CAD build for the part. Positions are in the model's coordinates, mm. Give positions to 0.01 mm unless a question says otherwise; leave off trailing zeros. Loops run counter-clockwise (first coordinate to the right, second up) from the corner with the lowest first, then second, coordinate; pieces in that order, holes last.
```python
from build123d import *

# Parameters (mm, degrees)
SKETCH1_R               = 25
BOSS_EXTRUDE1_DEPTH     = 3.5
SKETCH3_R               = 8.75
BOSS_EXTRUDE2_DEPTH     = 4
SKETCH4_R               = 2.625
CUT_EXTRUDE1_DEPTH      = 3.5
CUT_EXTRUDE2_DEPTH      = 10
CUT_EXTRUDE3_DEPTH      = 26
CUT_EXTRUDE3_DEPTH_BACK = 26
CUT_EXTRUDE4_DEPTH      = 26
CUT_EXTRUDE4_DEPTH_BACK = 26
SKETCH11_R              = 25
CUT_EXTRUDE5_DEPTH      = 3
BOSS_EXTRUDE3_DEPTH     = 3
SKETCH13_R              = 8.75
SKETCH13_R_2            = 2.55
BOSS_EXTRUDE4_DEPTH     = 3
SKETCH16_R              = 25
SKETCH16_R_2            = 2.625
BOSS_EXTRUDE5_DEPTH     = 2.5
SKETCH17_R              = 25
SKETCH17_R_2            = 8.75
CUT_EXTRUDE6_DEPTH      = 0.75
CUT_EXTRUDE7_DEPTH      = 1
SKETCH19_R              = 8.75
SKETCH19_R_2            = 3.5
CUT_EXTRUDE8_DEPTH      = 20
SKETCH20_R              = 6.415433717
CUT_EXTRUDE9_DEPTH      = 10
SKETCH22_R              = 3.5
CUT_EXTRUDE10_DEPTH     = 0.5


with BuildPart() as part:
    # Sketch1 → Boss-Extrude1 (new body)
    with BuildSketch(Plane(origin=(0, 0, 0), x_dir=(1, 0, 0), z_dir=(0, 1, 0))):
        Circle(SKETCH1_R)
    extrude(amount=BOSS_EXTRUDE1_DEPTH)

    # Sketch3 → Boss-Extrude2 (add)
    with BuildSketch(Plane(origin=(0, 3.5, 0), x_dir=(1, 0, 0), z_dir=(0, 1, 0))):
        Circle(SKETCH3_R)
    extrude(amount=BOSS_EXTRUDE2_DEPTH)

    # Sketch4 → Cut-Extrude1 (cut)
    with BuildSketch(Plane(origin=(0, 3.5, 0), x_dir=(1, 0, 0), z_dir=(0, 1, 0))):
        with Locations((0, 18.5)):
            Circle(SKETCH4_R)
        with Locations((13.081475452, 13.081475452)):
            Circle(SKETCH4_R)
        with Locations((18.5, 0)):
            Circle(SKETCH4_R)
        with Locations((13.081475452, -13.081475452)):
            Circle(SKETCH4_R)
        with Locations((0, -18.5)):
            Circle(SKETCH4_R)
        with Locations((-13.081475452, -13.081475452)):
            Circle(SKETCH4_R)
        with Locations((-18.5, 0)):
            Circle(SKETCH4_R)
        with Locations((-13.081475452, 13.081475452)):
            Circle(SKETCH4_R)
    extrude(amount=-CUT_EXTRUDE1_DEPTH, mode=Mode.SUBTRACT)

    # Sketch7 → Cut-Extrude2 (cut)
    with BuildSketch(Plane.XZ):
        with BuildLine():
            Line((1.9, 1.700735135), (1.9, -1.700735135))
            ThreePointArc((1.9, -1.700735135), (-2.55, 0), (1.9, 1.700735135))
        make_face()
    extrude(amount=-CUT_EXTRUDE2_DEPTH, mode=Mode.SUBTRACT)

    # Sketch8 → Cut-Extrude3 (cut, two sides)
    with BuildSketch(Plane(origin=(0, 0, 0), x_dir=(0, 0, -1), z_dir=(1, 0, 0))) as cut_extrude3_sk:
        with BuildLine():
            Line((-2.5, 6), (2.5, 6))
            ThreePointArc((2.5, 6), (3.5, 5), (2.5, 4))
            Line((2.5, 4), (-2.5, 4))
            ThreePointArc((-2.5, 4), (-3.5, 5), (-2.5, 6))
        make_face()
    extrude(amount=CUT_EXTRUDE3_DEPTH, mode=Mode.SUBTRACT)
    extrude(cut_extrude3_sk.sketch, amount=-CUT_EXTRUDE3_DEPTH_BACK, mode=Mode.SUBTRACT)

    # Sketch9 → Cut-Extrude4 (cut, two sides)
    with BuildSketch(Plane.XY) as cut_extrude4_sk:
        with BuildLine():
            Line((-2.5, 6), (2.5, 6))
            ThreePointArc((2.5, 6), (3.5, 5), (2.5, 4))
            Line((2.5, 4), (-2.5, 4))
            ThreePointArc((-2.5, 4), (-3.5, 5), (-2.5, 6))
        make_face()
    extrude(amount=CUT_EXTRUDE4_DEPTH, mode=Mode.SUBTRACT)
    extrude(cut_extrude4_sk.sketch, amount=-CUT_EXTRUDE4_DEPTH_BACK, mode=Mode.SUBTRACT)

    # Sketch11 → Cut-Extrude5 (cut)
    with BuildSketch(Plane(origin=(0, 3.5, 0), x_dir=(1, 0, 0), z_dir=(0, 1, 0))):
        Circle(SKETCH11_R)
    extrude(amount=-CUT_EXTRUDE5_DEPTH, mode=Mode.SUBTRACT)

    # Sketch12 → Boss-Extrude3 (add)
    with BuildSketch(Plane(origin=(0, 0.5, 0), x_dir=(1, 0, 0), z_dir=(0, 1, 0))):
        Polygon((0.6, 0.6), (5, 0.6), (5, -0.6), (0.6, -0.6), (0.6, -5), (-0.6, -5), (-0.6, -0.6), (-5, -0.6), (-5, 0.6), (-0.6, 0.6), (-0.6, 5), (0.6, 5), align=None)
    extrude(amount=BOSS_EXTRUDE3_DEPTH)

    # Sketch13 → Boss-Extrude4 (add)
    with BuildSketch(Plane(origin=(0, 0.5, 0), x_dir=(1, 0, 0), z_dir=(0, 1, 0))):
        Circle(SKETCH13_R)
        Circle(SKETCH13_R_2, mode=Mode.SUBTRACT)
    extrude(amount=BOSS_EXTRUDE4_DEPTH)

    # Sketch15 → Revolve1 (revolve)
    with BuildSketch(Plane.XY):
        Polygon((0, 13.5), (-8.75, 7.5), (0, 7.5), align=None)
    revolve(axis=Axis((0, -5.481339273, 0), (0, 1, 0)))

    # Sketch16 → Boss-Extrude5 (add)
    with BuildSketch(Plane.XZ):
        Circle(SKETCH16_R)
        with Locations((13.081475452, 13.081475452)):
            Circle(SKETCH16_R_2, mode=Mode.SUBTRACT)
        with Locations((0, 18.5)):
            Circle(SKETCH16_R_2, mode=Mode.SUBTRACT)
        with Locations((-13.081475452, 13.081475452)):
            Circle(SKETCH16_R_2, mode=Mode.SUBTRACT)
        with Locations((-18.5, 0)):
            Circle(SKETCH16_R_2, mode=Mode.SUBTRACT)
        with Locations((-13.081475452, -13.081475452)):
            Circle(SKETCH16_R_2, mode=Mode.SUBTRACT)
        with Locations((0, -18.5)):
            Circle(SKETCH16_R_2, mode=Mode.SUBTRACT)
        with Locations((13.081475452, -13.081475452)):
            Circle(SKETCH16_R_2, mode=Mode.SUBTRACT)
        with Locations((18.5, 0)):
            Circle(SKETCH16_R_2, mode=Mode.SUBTRACT)
        with BuildLine():
            Line((1.9, 1.700735135), (1.9, -1.700735135))
            ThreePointArc((1.9, -1.700735135), (-2.55, 0), (1.9, 1.700735135))
        make_face(mode=Mode.SUBTRACT)
    extrude(amount=BOSS_EXTRUDE5_DEPTH)

    # Sketch17 → Cut-Extrude6 (cut)
    with BuildSketch(Plane(origin=(0, 0.5, 0), x_dir=(1, 0, 0), z_dir=(0, 1, 0))):
        Circle(SKETCH17_R)
        Circle(SKETCH17_R_2, mode=Mode.SUBTRACT)
    extrude(amount=-CUT_EXTRUDE6_DEPTH, mode=Mode.SUBTRACT)

    # Sketch18 → Cut-Extrude7 (cut)
    with BuildSketch(Plane.XZ.offset(-0.5)):
        with BuildLine():
            Line((1.9, 1.700735135), (1.9, -1.700735135))
            ThreePointArc((1.9, -1.700735135), (-2.55, 0), (1.9, 1.700735135))
        make_face()
    extrude(amount=-CUT_EXTRUDE7_DEPTH, mode=Mode.SUBTRACT)

    # Sketch19 → Cut-Extrude8 (cut)
    with BuildSketch(Plane(origin=(0, -0.25, 0), x_dir=(1, 0, 0), z_dir=(0, 1, 0))):
        Circle(SKETCH19_R)
        Circle(SKETCH19_R_2, mode=Mode.SUBTRACT)
    extrude(amount=CUT_EXTRUDE8_DEPTH, mode=Mode.SUBTRACT)

    # Sketch20 → Cut-Extrude9 (cut)
    with BuildSketch(Plane.XZ.offset(-6)):
        Circle(SKETCH20_R)
    extrude(amount=-CUT_EXTRUDE9_DEPTH, mode=Mode.SUBTRACT)

    # Sketch22 → Cut-Extrude10 (cut)
    with BuildSketch(Plane(origin=(0, 4, 0), x_dir=(1, 0, 0), z_dir=(0, 1, 0))):
        Circle(SKETCH22_R)
    extrude(amount=-CUT_EXTRUDE10_DEPTH, mode=Mode.SUBTRACT)

    # Sketch23 → Cut-Revolve3 (revolve, cut)
    with BuildSketch(Plane(origin=(0, 0, 0), x_dir=(0, 0, -1), z_dir=(1, 0, 0))):
        Polygon((3.5, 1.625), (0.6, 3.5), (3.5, 3.5), align=None)
    revolve(axis=Axis((0, -5.481339273, 0), (0, 1, 0)), mode=Mode.SUBTRACT)


solid = part.part
```
1. Probe line 1 along X through (y, z) = (-1.5, 0) (3 decimals); line 2 along Z through (x, y) = (0, -0.75) (3 decimals); line 3 along X through (y, z) = (0.35, 0). List the from-to ranges inside material, lowest first.
Responses:
line 1: x = -25 to -21.125, -15.875 to -2.55, 1.9 to 15.875, 21.125 to 25
line 2: z = -25 to -21.125, -15.875 to -2.55, 2.55 to 15.875, 21.125 to 25
line 3: x = -3.5 to -2.55, 1.9 to 3.5
2. Saw through at D-D, the plane x = -18.5. List the corners of the cut face in (y, z) (3 decimals), and give its area (3 significant figures).
Responses:
outline: (-2.5, -16.815) - (-0.25, -16.815) - (-0.25, -2.625) - (-2.5, -2.625) - close; (-2.5, 2.625) - (-0.25, 2.625) - (-0.25, 16.815) - (-2.5, 16.815) - close
area: 63.9 mm2
3. Saw through at C-C, the plane z = -18.5. List the corners of the cut face in (x, y) (3 decimals), and give its area (3 significant figures).
Responses:
outline: (-16.815, -2.5) - (-2.625, -2.5) - (-2.625, -0.25) - (-16.815, -0.25) - close; (2.625, -2.5) - (16.815, -2.5) - (16.815, -0.25) - (2.625, -0.25) - close
area: 63.9 mm2
4. Saw through at B-B, the plane x = 0. List the corners of the cut face in (y, z) (3 decimals).
Responses:
outline: (-2.5, -25) - (-0.25, -25) - (-0.25, -21.125) - (-2.5, -21.125) - close; (-2.5, -15.875) - (-0.25, -15.875) - (-0.25, -3.5) - (1.625, -3.5) - (3.5, -0.6) - (3.5, 0.6) - (1.625, 3.5) - (-0.25, 3.5) - (-0.25, 15.875) - (-2.5, 15.875) - (-2.5, 2.55) - (1.5, 2.55) - (1.5, -2.55) - (-2.5, -2.55) - close; (-2.5, 21.125) - (-0.25, 21.125) - (-0.25, 25) - (-2.5, 25) - close
5. Drop flat-ended pins along their axis: pin 1 (1.2 mm diameter, centred on y = -1, z = 0.5, fed in from -X); pin 2 (2 mm diameter, centred on x = 0, y = 1.5, fed in from -Z); pin 3 (3 mm diameter, centred on y = -1, z = -20, fed in from +X); pin 4 (2 mm diameter, centred on y = 2, z = 1.5, fed in from -X). Give the stop position or say it passes through.
Responses:
pin 1: stops at x = -25
pin 2: stops at z = -3.5
pin 3: stops at x = 16.82
pin 4: stops at x = -3.45
6. Pull direction X, two halves, no side cores. Call faces 1 (the face through (0, -0.25, 5)), 2 (the face through (2, 2, -0.6)), 3 (the face through (3.233, 0.674, 1.341)): released by +X, released by -X, zero draft, split by the parting line, or undercut.
Responses:
face 1: zero draft
face 2: undercut
face 3: split by the parting line
7. Saw through at A-A, the plane z = 0. List the corners of the cut face in (x, y) (3 decimals), and give its area (3 significant figures).
Responses:
outline: (-25, -2.5) - (-21.125, -2.5) - (-21.125, -0.25) - (-25, -0.25) - close; (-15.875, -2.5) - (-2.55, -2.5) - (-2.55, 1.5) - (1.9, 1.5) - (1.9, -2.5) - (15.875, -2.5) - (15.875, -0.25) - (3.5, -0.25) - (3.5, 1.625) - (0.6, 3.5) - (-0.6, 3.5) - (-3.5, 1.625) - (-3.5, -0.25) - (-15.875, -0.25) - close; (21.125, -2.5) - (25, -2.5) - (25, -0.25) - (21.125, -0.25) - close
area: 91.9 mm2
